Design review of the part built by this model. Coordinates are the model's own, in mm. Coordinates: 2 decimals unless noted, no trailing zeros. Write each loop counter-clockwise with the first axis right and the second up, starting at its lowest first coordinate (ties: lowest second). Pieces come first, ordered by that corner, then holes.
Q1. Insertion check: pin 1 (11.5 mm diameter, centred on x = -8.65, y = 33.44, fed in from -Z); pin 2 (1.5 mm diameter, centred on x = -28, z = 2.5, fed in from +Y). Each pin has a flat end and moves straight along its axis. Give the tip position at first contact, or say it passes through.
Q2. Take a section at C-C (x = 4). Give the boundary of the cut face in (y, z).
Q3. For probe 1 along X at (y, z) = (-17.5, 3.5); probe 2 along X at (y, z) = (2.5, 1.85); probe 3 along X at (y, z) = (-1, 1), list the stretches that pass through material, from the lowest coordinate up.
Q4. Take a section at B-B (x = -28). Give the boundary of the cut face in (y, z), and give its area (3 significant figures).
Q5. Take a section at A-A (z = 1.1). Give the boundary of the cut face in (x, y) (3 decimals), and give its area (3 significant figures).
```python
from build123d import *

# Parameters (mm, degrees)
SKETCH_1_R          = 13.625
SKETCH_1_R_2        = 9.5
EXTRUDE_1_DEPTH     = 4
SKETCH_2_R          = 2
CUT_EXTRUDE_1_DEPTH = 4


with BuildPart() as part:
    # 草图1 → 凸台-拉伸1 (new body)
    with BuildSketch(Plane.XY):
        with BuildLine():
            ThreePointArc((-9.939636128, -36.721524578), (0, -42.437612957), (9.939636128, -36.721524578))
            ThreePointArc((9.939636128, -36.721524578), (13.271431273, -34.0328785), (17.547256679, -34.24965882))
            ThreePointArc((17.547256679, -34.24965882), (28.948423675, -33.03169993), (33.629925771, -22.564915761))
            ThreePointArc((33.629925771, -22.564915761), (34.745058151, -18.431375342), (38.331693845, -16.093487189))
            ThreePointArc((38.331693845, -16.093487189), (46.839533428, -8.40669993), (44.474726808, 2.81282423))
            ThreePointArc((44.474726808, 2.81282423), (42.947253757, 6.812387043), (44.474726808, 10.811949856))
            ThreePointArc((44.474726808, 10.811949856), (46.839533428, 22.031474016), (38.331693845, 29.718261275))
            ThreePointArc((38.331693845, 29.718261275), (34.745058151, 32.056149427), (33.629925771, 36.189689846))
            ThreePointArc((33.629925771, 36.189689846), (28.948423675, 46.656474016), (17.547256679, 47.874432905))
            ThreePointArc((17.547256679, 47.874432905), (13.271431273, 47.657652585), (9.939636128, 50.346298663))
            ThreePointArc((9.939636128, 50.346298663), (0, 56.062387043), (-9.939636128, 50.346298663))
            ThreePointArc((-9.939636128, 50.346298663), (-13.271431273, 47.657652585), (-17.547256679, 47.874432905))
            ThreePointArc((-17.547256679, 47.874432905), (-28.948423675, 46.656474016), (-33.629925771, 36.189689846))
            ThreePointArc((-33.629925771, 36.189689846), (-34.745058151, 32.056149427), (-38.331693845, 29.718261275))
            ThreePointArc((-38.331693845, 29.718261275), (-46.839533428, 22.031474016), (-44.474726808, 10.811949856))
            ThreePointArc((-44.474726808, 10.811949856), (-42.947253757, 6.812387043), (-44.474726808, 2.81282423))
            ThreePointArc((-44.474726808, 2.81282423), (-46.839533428, -8.40669993), (-38.331693845, -16.093487189))
            ThreePointArc((-38.331693845, -16.093487189), (-34.745058151, -18.431375342), (-33.629925771, -22.564915761))
            ThreePointArc((-33.629925771, -22.564915761), (-28.948423675, -33.03169993), (-17.547256679, -34.24965882))
            ThreePointArc((-17.547256679, -34.24965882), (-13.271431273, -34.0328785), (-9.939636128, -36.721524578))
        make_face()
        with Locations((0, 6.812387043)):
            Circle(SKETCH_1_R, mode=Mode.SUBTRACT)
        with Locations((-8.652475842, -19.817195414)):
            Circle(SKETCH_1_R_2, mode=Mode.SUBTRACT)
        with Locations((-28, 6.812387043)):
            Circle(SKETCH_1_R_2, mode=Mode.SUBTRACT)
        with Locations((-8.652475842, 33.441969499)):
            Circle(SKETCH_1_R_2, mode=Mode.SUBTRACT)
        with Locations((22.652475842, 23.270374107)):
            Circle(SKETCH_1_R_2, mode=Mode.SUBTRACT)
        with Locations((22.652475842, -9.645600022)):
            Circle(SKETCH_1_R_2, mode=Mode.SUBTRACT)
    extrude(amount=EXTRUDE_1_DEPTH)

    # 草图2 → 切除-拉伸1 (cut)
    with BuildSketch(Plane.XY.offset(4)):
        with Locations((13.625, 6.812387043)):
            Circle(SKETCH_2_R)
    extrude(amount=-CUT_EXTRUDE_1_DEPTH, mode=Mode.SUBTRACT)


solid = part.part
```
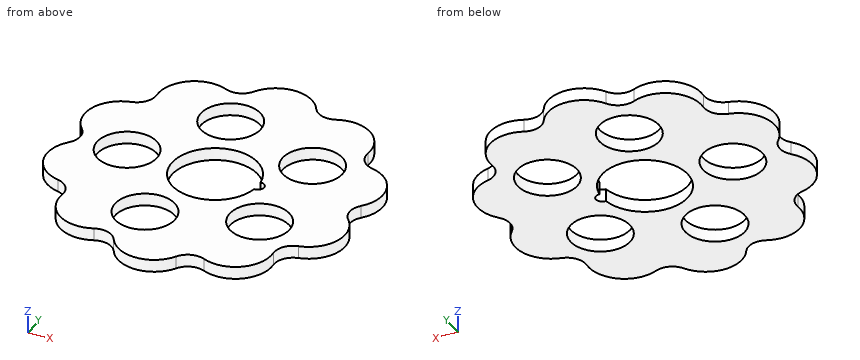
Response:
1. pin 1: passes through
1. pin 2: stops at y = 47.68
2. outline: (-41.72, 0) - (-6.21, 0) - (-6.21, 4) - (-41.72, 4) - close; (19.84, 0) - (55.34, 0) - (55.34, 4) - (19.84, 4) - close
3. probe 1: x = -35.58 to -17.87, 0.56 to 17.31, 28 to 35.58
3. probe 2: x = -44.74 to -36.46, -19.54 to -12.92, 12.92 to 44.74
3. probe 3: x = -46.74 to -33.41, -22.59 to -11.16, 11.16 to 18.72, 26.59 to 46.74
4. outline: (-33.65, 0) - (-2.69, 0) - (-2.69, 4) - (-33.65, 4) - close; (16.31, 0) - (47.28, 0) - (47.28, 4) - (16.31, 4) - close
4. area: 248 mm2
5. outline: (-44.475, 2.813) arc R11.5 ccw to (-38.332, -16.093) arc R6 cw to (-33.63, -22.565) arc R11.5 ccw to (-17.547, -34.25) arc R6 cw to (-9.94, -36.722) arc R11.5 ccw to (9.94, -36.722) arc R6 cw to (17.547, -34.25) arc R11.5 ccw to (33.63, -22.565) arc R6 cw to (38.332, -16.093) arc R11.5 ccw to (44.475, 2.813) arc R6 cw to (44.475, 10.812) arc R11.5 ccw to (38.332, 29.718) arc R6 cw to (33.63, 36.19) arc R11.5 ccw to (17.547, 47.874) arc R6 cw to (9.94, 50.346) arc R11.5 ccw to (-9.94, 50.346) arc R6 cw to (-17.547, 47.874) arc R11.5 ccw to (-33.63, 36.19) arc R6 cw to (-38.332, 29.718) arc R11.5 ccw to (-44.475, 10.812) arc R6 cw to start; hole circle Ø19 at (-28, 6.812); hole circle Ø19 at (-8.652, -19.817); hole circle Ø19 at (-8.652, 33.442); hole circle Ø19 at (22.652, -9.646); hole circle Ø19 at (22.652, 23.27); hole (13.478, 4.818) arc R2 ccw (long way) to (13.478, 8.807) arc R13.625 ccw (long way) to start
5. area: 4,820 mm2
